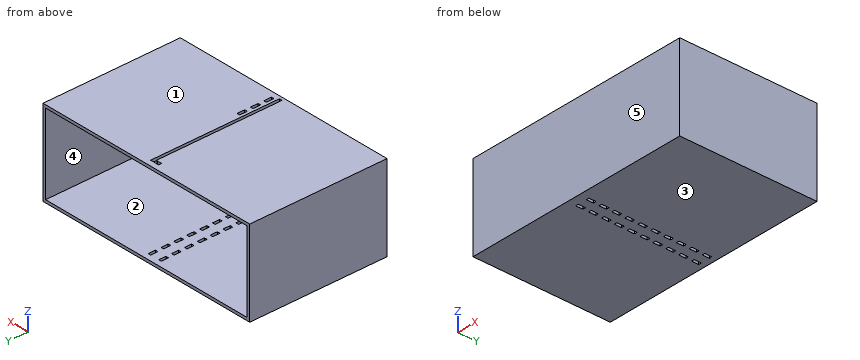
from build123d import *

# Parameters (mm, degrees)
SKETCH1_W           = 508
SKETCH1_H           = 190.5
BOSS_EXTRUDE1_DEPTH = 6.35
SKETCH2_W           = 508
SKETCH2_H           = 190.5
SKETCH2_W_2         = 495.3
SKETCH2_H_2         = 177.8
BOSS_EXTRUDE2_DEPTH = 298.45
SKETCH3_W           = 6.35
SKETCH3_H           = 16.933333333
SKETCH3_H_2         = 16.933333334
CUT_EXTRUDE1_DEPTH  = 12.7
SKETCH4_W           = 6.35
SKETCH4_H           = 15.875
CUT_EXTRUDE2_DEPTH  = 6.35


with BuildPart() as part:
    # Sketch1 → Boss-Extrude1 (new body)
    with BuildSketch(Plane(origin=(0, 0, 0), x_dir=(1, 0, 0), z_dir=(0, 1, 0))):
        Rectangle(SKETCH1_W, SKETCH1_H)
    extrude(amount=BOSS_EXTRUDE1_DEPTH)

    # Sketch2 → Boss-Extrude2 (add)
    with BuildSketch(Plane(origin=(0, 6.35, 0), x_dir=(1, 0, 0), z_dir=(0, 1, 0))):
        Rectangle(SKETCH2_W, SKETCH2_H)
        Rectangle(SKETCH2_W_2, SKETCH2_H_2, mode=Mode.SUBTRACT)
    extrude(amount=BOSS_EXTRUDE2_DEPTH)

    # Sketch3 → Cut-Extrude1 (cut)
    with BuildSketch(Plane.XY.offset(95.25)):
        with BuildLine():
            Line((-3.302, 283.21), (-3.302, 6.35))
            Line((-3.302, 6.35), (3.302, 6.35))
            Line((3.302, 6.35), (3.302, 292.354))
            Line((3.302, 292.354), (-16.256, 292.354))
            Line((-16.256, 292.354), (-16.256, 285.75))
            Line((-16.256, 285.75), (-5.842, 285.75))
            ThreePointArc((-5.842, 285.75), (-4.045948776, 285.006051224), (-3.302, 283.21))
        make_face()
        with Locations((12.827, 80.433333334)):
            Rectangle(SKETCH3_W, SKETCH3_H)
        with Locations((12.827, 50.8)):
            Rectangle(SKETCH3_W, SKETCH3_H_2)
        with Locations((12.827, 21.166666667)):
            Rectangle(SKETCH3_W, SKETCH3_H)
    extrude(amount=-CUT_EXTRUDE1_DEPTH, mode=Mode.SUBTRACT)

    # Sketch4 → Cut-Extrude2 (cut)
    with BuildSketch(Plane.XY.offset(-88.9)):
        with Locations((-19.431, 284.1625)):
            Rectangle(SKETCH4_W, SKETCH4_H)
        with Locations((-19.431, 255.5875)):
            Rectangle(SKETCH4_W, SKETCH4_H)
        with Locations((-19.431, 227.0125)):
            Rectangle(SKETCH4_W, SKETCH4_H)
        with Locations((-19.431, 198.4375)):
            Rectangle(SKETCH4_W, SKETCH4_H)
        with Locations((-19.431, 169.8625)):
            Rectangle(SKETCH4_W, SKETCH4_H)
        with Locations((-19.431, 141.2875)):
            Rectangle(SKETCH4_W, SKETCH4_H)
        with Locations((-19.431, 112.7125)):
            Rectangle(SKETCH4_W, SKETCH4_H)
        with Locations((-19.431, 84.1375)):
            Rectangle(SKETCH4_W, SKETCH4_H)
        with Locations((-19.431, 55.5625)):
            Rectangle(SKETCH4_W, SKETCH4_H)
        with Locations((-19.431, 26.9875)):
            Rectangle(SKETCH4_W, SKETCH4_H)
    cut_extrude2 = extrude(amount=-CUT_EXTRUDE2_DEPTH, mode=Mode.SUBTRACT)

    # Mirror1: Cut-Extrude2 across plane
    add(cut_extrude2.mirror(Plane.ZY.offset(6.477)), mode=Mode.SUBTRACT)


solid = part.part
Part model, mm, in its own coordinate system. Face numbers are marked on the shaded views. A direction names the side the tool comes from. Give positions to 0.01 mm unless a question says otherwise; leave off trailing zeros. Order: outer loops, then holes, each group sorted by start corner. A loop starts at its lowest first (then second) coordinate and runs counter-clockwise, first axis right, second up. Notation, with made-up numbers: (16, 21.5) -> (36, 21.5) arc R27 ccw to (36, 50.5) -> close; hole circle Ø9 at (1, 62.25). An arc over 180 degrees is marked (long way). Use one line per item in the form item = value.
(1) Saw through at A-A (y = 142). Write the cut outline in (x, z), then the cut area to 3 significant figures.
Solution:
outline = (-254, -95.25) -> (-22.61, -95.25) -> (-22.61, -88.9) -> (-247.65, -88.9) -> (-247.65, 88.9) -> (-3.3, 88.9) -> (-3.3, 95.25) -> (-254, 95.25) -> close; (-16.26, -95.25) -> (3.3, -95.25) -> (3.3, -88.9) -> (-16.26, -88.9) -> close; (3.3, 88.9) -> (247.65, 88.9) -> (247.65, -88.9) -> (9.65, -88.9) -> (9.65, -95.25) -> (254, -95.25) -> (254, 95.25) -> (3.3, 95.25) -> close
area = 8,590 mm²
(2) Saw through at C-C (x = -96.5). Write the cut outline in (y, z), then the cut area to 3 significant figures.
Solution:
outline = (0, -95.25) -> (304.8, -95.25) -> (304.8, -88.9) -> (6.35, -88.9) -> (6.35, 88.9) -> (304.8, 88.9) -> (304.8, 95.25) -> (0, 95.25) -> close
area = 5,000 mm²
(3) Drill centre lines: line 1 (X direction, y = 229, z = -17); line 2 (Z direction, x = -38.5, y = 227); line 3 (Y direction, x = 165, z = -71). Where is each one in solid material? Low to high. Write a range as from..to.
Solution:
line_1 = -254..-247.65, 247.65..254
line_2 = -95.25..-88.9, 88.9..95.25
line_3 = 0..6.35
(4) Pull direction Z, two halves, no side cores. Call the marked faces 3, 4 and 5: +Z half, -Z half, draft (parallel to the pull), parting line (faces both ways), or undercut.
Solution:
face_3 = -Z half
face_4 = undercut
face_5 = draft
(5) Saw through at B-B (z = -55.5). Write the cut outline in (x, y).
Solution:
outline = (-254, 0) -> (254, 0) -> (254, 304.8) -> (247.65, 304.8) -> (247.65, 6.35) -> (-247.65, 6.35) -> (-247.65, 304.8) -> (-254, 304.8) -> close
(6) Tool access for the marked faces 1 and 2: list every direction of +Z, -Z, +X, -X, +Y, -Y with a clear straight run to the whole face (end or side of a thin tool).
Solution:
face_1 = +Z, +X, -X, +Y, -Y
face_2 = +Y
